Source: CAD feature listing. Evaluate the final solid. Frame: model axes, mm. A direction names the side the tool comes from. Coordinates: 2 decimals unless noted, no trailing zeros. Write each loop counter-clockwise with the first axis right and the second up, starting at its lowest first coordinate (ties: lowest second). Pieces come first, ordered by that corner, then holes. Notation, with made-up numbers: (6.5, 80.5) -> (64.5, 80.5) arc R22 cw to (64.5, 91.5) -> close; hole circle Ø5 at (-3, 37.25). An arc over 180 degrees is marked (long way). Write item = value, one per line.
from build123d import *

# Parameters (mm, degrees)
F0_W     = 100
F0_H     = 40
F1_DEPTH = 10
F3_DEPTH = 10
F4_R     = 2.25
F5_DEPTH = 40.001
F6_R     = 4.5
F7_DEPTH = 5.7


with BuildPart() as f1:
    # F0 (on Top) → F1 (new body)
    with BuildSketch(Plane.XY):
        with Locations((50, 20)):
            Rectangle(F0_W, F0_H)
    extrude(amount=F1_DEPTH)

    # F2 (on face) → F3 (join)
    with BuildSketch(Plane.XZ):
        with BuildLine():
            Line((39.282996, 35), (39.282996, 0))
            Line((39.282996, 0), (60.717004, 0))
            Line((60.717004, 0), (60.717004, 35))
            ThreePointArc((60.717004, 35), (50, 45.717004), (39.282996, 35))
        make_face()
    extrude(amount=-F3_DEPTH)

    # F4 (on face) → F5 (cut, through all)
    with BuildSketch(Plane.XZ):
        with Locations((50, 35)):
            Circle(F4_R)
    extrude(amount=-F5_DEPTH, mode=Mode.SUBTRACT)

    # F6 (on face) → F7 (cut)
    with BuildSketch(Plane.XZ):
        with Locations((50, 35)):
            Circle(F6_R)
    extrude(amount=-F7_DEPTH, mode=Mode.SUBTRACT)


solid = f1.part
1) Cut plane A-A, the plane x = 50. Output: boundary loops of the cut face in (y, z).
Answer block:
outline = (0, 0) -> (40, 0) -> (40, 10) -> (10, 10) -> (10, 32.75) -> (5.7, 32.75) -> (5.7, 30.5) -> (0, 30.5) -> close; (0, 39.5) -> (5.7, 39.5) -> (5.7, 37.25) -> (10, 37.25) -> (10, 45.72) -> (0, 45.72) -> close
2) Cut plane C-C, the plane y = 24.5. Output: boundary loops of the cut face in (x, z).
Answer block:
outline = (0, 0) -> (100, 0) -> (100, 10) -> (0, 10) -> close
3) Cut plane B-B, the plane z = 22.5. Output: boundary loops of the cut face in (x, y).
Answer block:
outline = (39.28, 0) -> (60.72, 0) -> (60.72, 10) -> (39.28, 10) -> close
4) Reachability of faces 4 (the flat face through (39.283, 5, 23)), 5 (the flat face through (52, 5.7, 33)), 6 (the flat face through (50, 10, 28)), 7 (the flat face through (50, 0, 11)) from +Z, -Z, +X, -X, +Y, -Y: full face, straight path, thin tool, end or side. Return the list, or none.
Answer block:
face_4 = +Z, -X, +Y, -Y
face_5 = -Y
face_6 = +Z, +X, -X, +Y
face_7 = +Z, -Z, +X, -X, -Y
5) Pull-direction query (Z, two-part tool) for faces 1 (the cylindrical face through (52.08, 2.81, 31.01)), 2 (the flat face through (49, 20, 10)), 3 (the flat face through (60.717, 5, 22)); classes: +Z half, -Z half, draft (parallel to the pull), parting line (faces both ways), or undercut.
Answer block:
face_1 = undercut
face_2 = +Z half
face_3 = draft
6) First-contact query: pin 1 Ø8 at (y, z) = (7, 28) entering from +X; pin 2 Ø10 at (x, y) = (33, 10.5) entering from +Z; pin 3 Ø17 at (x, z) = (48.5, 24.5) entering from +Y. Flat tips, straight axial feed; report the tip coordinate or a pass-through.
Answer block:
pin_1 = 60.72
pin_2 = 10
pin_3 = 10
7) Material intervals for probe 1 along Z at (x, y) = (50, 6.8); probe 2 along Z at (x, y) = (50, 2.6); probe 3 along Z at (x, y) = (48.5, 20), sorted ascending. Write a range as [from, to].
Answer block:
probe_1 = [0, 32.75], [37.25, 45.72]
probe_2 = [0, 30.5], [39.5, 45.72]
probe_3 = [0, 10]
